from build123d import *

# Parameters (mm, degrees)
SKETCH_1_W      = 30
SKETCH_1_H      = 50
EXTRUDE_1_DEPTH = 10
SKETCH_2_W      = 30
SKETCH_2_H      = 50
EXTRUDE_2_DEPTH = 20
EXTRUDE_2_DRAFT = -30
EXTRUDE_3_DEPTH = 35


with BuildPart() as part:
    # 草图1 → 凸台-拉伸1 (new body)
    with BuildSketch(Plane.XY):
        Rectangle(SKETCH_1_W, SKETCH_1_H)
    extrude(amount=EXTRUDE_1_DEPTH)


with BuildPart() as extrude_2_tool:
    # 草图2 → 凸台-拉伸2 (with draft: the straight prism first)
    with BuildSketch(Plane.XY.offset(10)):
        Rectangle(SKETCH_2_W, SKETCH_2_H)
    extrude(amount=EXTRUDE_2_DEPTH)
    # 凸台-拉伸2: the draft: its side faces are tilted about the plane it starts from
    extrude_2_sides = [extrude_2_tool.faces().sort_by_distance(p)[0] for p in [
        (15, 0, 20),
        (0, 25, 20),
        (-15, 0, 20),
        (0, -25, 20),
    ]]
    draft(extrude_2_sides, Plane.XY.offset(10), EXTRUDE_2_DRAFT)


with BuildPart() as part_1:
    add(part.part)

    # 凸台-拉伸2: add extrude_2_tool
    add(extrude_2_tool.part)

    # 草图3 → 凸台-拉伸3 (add, symmetric)
    with BuildSketch(Plane(origin=(0, 0, 0), x_dir=(0, 0, -1), z_dir=(1, 0, 0))):
        with BuildLine():
            Line((-30, 36.547005384), (-30, -36.547005384))
            ThreePointArc((-30, -36.547005384), (-112.063957994, 0), (-30, 36.547005384))
        make_face()
    extrude(amount=EXTRUDE_3_DEPTH, both=True)


solid = part_1.part
Read the model definition and answer for the solid it produces. Units are mm, in the model's axes. A direction names the side the tool comes from. Coordinates: 2 decimals unless noted, no trailing zeros. Order: outer loops, then holes, each group sorted by start corner. A loop starts at its lowest first (then second) coordinate and runs counter-clockwise, first axis right, second up. Notation, with made-up numbers: (88, 59) -> (137, 59) arc R18 cw to (137, 83) -> close; hole circle Ø4 at (34, 72.25). An arc over 180 degrees is marked (long way). Answer as a JSON object with one key per item and string values.
1) Consider line 1 along X through (y, z) = (-15.5, 6); line 2 along Y through (x, z) = (0.5, 64.5); line 3 along Y through (x, z) = (-8, 90.5). Determine where each line is inside the solid, lowest interval first. Write a range as from..to.
Model answer:
{"line 1": "x = -15..15", "line 2": "y = -49.14..49.14", "line 3": "y = -40.69..40.69"}
2) A cutting plane is placed at A-A, the plane y = 0. Determine the outline of the cut face in (x, z), plus the area to 3 significant figures.
Model answer:
{"outline": "(-35, 30) -> (-26.55, 30) -> (-15, 10) -> (-15, 0) -> (15, 0) -> (15, 10) -> (26.55, 30) -> (35, 30) -> (35, 112.06) -> (-35, 112.06) -> close", "area": "6,880 mm²"}
3) A cutting plane is placed at D-D, the plane z = 27. Determine the outline of the cut face in (x, y).
Model answer:
{"outline": "(-24.81, -34.81) -> (24.81, -34.81) -> (24.81, 34.81) -> (-24.81, 34.81) -> close"}
4) A cutting plane is placed at B-B, the plane x = 6. Determine the outline of the cut face in (y, z), plus the area to 3 significant figures.
Model answer:
{"outline": "(-36.55, 30) -> (-25, 10) -> (-25, 0) -> (25, 0) -> (25, 10) -> (36.55, 30) arc R49.17 ccw (long way) to start", "area": "8,500 mm²"}
5) A tool of negligible diameter and unlimited length cuts with its end or side. For faces 1 (the face through (0, 0, 0)), 2 (the face through (0, 25, 5)), 3 (the face through (0, -25, 5)), 4 (the face through (-31, 1, 30)), 5 (the face through (31, 1, 30)), from which of +Z, -Z, +X, -X, +Y, -Y can it reach the whole face along a straight path? Write none if from no direction.
Model answer:
{"face 1": "-Z, +X, -X, +Y, -Y", "face 2": "-Z, +X, -X, +Y", "face 3": "-Z, +X, -X, -Y", "face 4": "-Z, -X, +Y, -Y", "face 5": "-Z, +X, +Y, -Y"}
6) A cutting plane is placed at C-C, the plane y = -34. Determine the outline of the cut face in (x, z).
Model answer:
{"outline": "(-35, 30) -> (-26.55, 30) -> (-24, 25.59) -> (24, 25.59) -> (26.55, 30) -> (35, 30) -> (35, 98.41) -> (-35, 98.41) -> close"}
7) Each of these flat-tipped pins is pushed along its axis until it touches: pin 1 (5 mm diameter, centred on y = 9.5, z = 5.5, fed in from +X); pin 2 (4 mm diameter, centred on x = -29, y = 10.5, fed in from -Z); pin 3 (6 mm diameter, centred on x = 27, z = 39, fed in from -Y); pin 4 (3 mm diameter, centred on x = 7, y = -22, fed in from -Z). Where does it stop, or does it pass through?
Model answer:
{"pin 1": "stops at x = 15", "pin 2": "stops at z = 30", "pin 3": "stops at y = -44.51", "pin 4": "stops at z = 0"}
